For this review, take the finished solid that the model builds, in its own axes (mm). A direction names the side the tool comes from. Round coordinates to 2 decimals unless told otherwise and drop trailing zeros. Order: outer loops, then holes, each group sorted by start corner. A loop starts at its lowest first (then second) coordinate and runs counter-clockwise, first axis right, second up. Notation, with made-up numbers: (69, 54.5) -> (81, 54.5) arc R23 ccw to (81, 86.5) -> close; hole circle Ø5 at (7.25, -7). An arc over 180 degrees is marked (long way). Answer in a Markdown table with one row per item.
```python
from build123d import *

# Parameters (mm, degrees)
F0_W     = 152.4
F0_H     = 114.3
F1_DEPTH = 152.4
F2_W     = 76.2
F2_H     = 30.254747
F3_DEPTH = 152.401
F2_W_2   = 38.1
F2_H_2   = 49.729511
F4_DEPTH = 152.401
F2_H_3   = 45.411082
F5_DEPTH = 152.401


with BuildPart() as f1:
    # F0 (on Front) → F1 (new body)
    with BuildSketch(Plane.XZ):
        Rectangle(F0_W, F0_H)
    extrude(amount=F1_DEPTH)

    # F2 (on face) → F3 (cut, through all)
    with BuildSketch(Plane.XZ.offset(152.4)):
        with Locations((0, 42.022627)):
            Rectangle(F2_W, F2_H)
    extrude(amount=-F3_DEPTH, mode=Mode.SUBTRACT)

    # F2 (on face) → F4 (cut, through all)
    with BuildSketch(Plane.XZ.offset(152.4)):
        with Locations((-57.15, -5.814755)):
            Rectangle(F2_W_2, F2_H_2)
    extrude(amount=-F4_DEPTH, mode=Mode.SUBTRACT)

    # F2 (on face) → F5 (cut, through all)
    with BuildSketch(Plane.XZ.offset(152.4)):
        with Locations((57.15, -3.655541)):
            Rectangle(F2_W_2, F2_H_3)
    extrude(amount=-F5_DEPTH, mode=Mode.SUBTRACT)


solid = f1.part
```
Q1. To check wall thickness, follow probe 1 along Z at (x, y) = (-54, -45.5); probe 2 along Z at (x, y) = (64.5, -116.5); probe 3 along X at (y, z) = (-66, 40). State the ranges of each line that lie inside material, in increasing order.
Answer key:
| item | result |
|---|---|
| probe 1 | z = -57.15 to -30.68, 19.05 to 57.15 |
| probe 2 | z = -57.15 to -26.36, 19.05 to 57.15 |
| probe 3 | x = -76.2 to -38.1, 38.1 to 76.2 |
Q2. Clearance check with flat-ended pins moving along their axes: pin 1 Ø25 at (y, z) = (-92.5, -11.5) entering from -X; pin 2 Ø1 at (y, z) = (-87, 12) entering from +X; pin 3 Ø8 at (x, y) = (12, -95.5) entering from +Z. State where each tip first meets the part, or that it passes through.
Answer key:
| item | result |
|---|---|
| pin 1 | stops at x = -38.1 |
| pin 2 | stops at x = 38.1 |
| pin 3 | stops at z = 26.9 |
Q3. The part is to be moulded in two halves that separate along Z. For faces 1 (the face through (38.1, -77, -4)), 2 (the face through (57, -75, 57.15)), 3 (the face through (-76.2, -75, -44)), say which applies: +Z half, -Z half, draft (parallel to the pull), parting line (faces both ways), or undercut.
Answer key:
| item | result |
|---|---|
| face 1 | undercut |
| face 2 | +Z half |
| face 3 | draft |
Q4. Take a section at B-B, the plane z = 39.5. Write out the cut boundary in (x, y).
Answer key:
| item | result |
|---|---|
| outline | (-76.2, -152.4) -> (-38.1, -152.4) -> (-38.1, 0) -> (-76.2, 0) -> close; (38.1, -152.4) -> (76.2, -152.4) -> (76.2, 0) -> (38.1, 0) -> close |
Q5. Take a section at C-C, the plane y = -29.5. Write out the cut boundary in (x, z).
Answer key:
| item | result |
|---|---|
| outline | (-76.2, -57.15) -> (76.2, -57.15) -> (76.2, -26.36) -> (38.1, -26.36) -> (38.1, 19.05) -> (76.2, 19.05) -> (76.2, 57.15) -> (38.1, 57.15) -> (38.1, 26.9) -> (-38.1, 26.9) -> (-38.1, 57.15) -> (-76.2, 57.15) -> (-76.2, 19.05) -> (-38.1, 19.05) -> (-38.1, -30.68) -> (-76.2, -30.68) -> close |
Q6. Take a section at A-A, the plane x = 63. Write out the cut boundary in (y, z), then the cut area to 3 significant figures.
Answer key:
| item | result |
|---|---|
| outline | (-152.4, -57.15) -> (0, -57.15) -> (0, -26.36) -> (-152.4, -26.36) -> close; (-152.4, 19.05) -> (0, 19.05) -> (0, 57.15) -> (-152.4, 57.15) -> close |
| area | 10,500 mm^2 |
Q7. Take a section at D-D, the plane z = -16. Write out the cut boundary in (x, y), then the cut area to 3 significant figures.
Answer key:
| item | result |
|---|---|
| outline | (-38.1, -152.4) -> (38.1, -152.4) -> (38.1, 0) -> (-38.1, 0) -> close |
| area | 11,600 mm^2 |
Q8. Tool access review of faces 4 (the face through (57, -77, 19.05)), 5 (the face through (-57, -77, 19.05)), 6 (the face through (-38.1, -77, 42)): name each direction out of +Z, -Z, +X, -X, +Y, -Y from which nothing blocks a thin tool from reaching the whole face with its end or side.
Answer key:
| item | result |
|---|---|
| face 4 | +X, +Y, -Y |
| face 5 | -X, +Y, -Y |
| face 6 | +Z, +Y, -Y |
